from build123d import *

# Parameters (mm, degrees)
SALIENTE_EXTRUIR1_DEPTH = 6


with BuildPart() as part:
    # Croquis1 → Saliente-Extruir1 (new body)
    with BuildSketch(Plane.XY):
        with BuildLine():
            Line((-283.764, 132.5), (-132.5, 132.5))
            Line((-132.5, 132.5), (-132.5, 283.764))
            ThreePointArc((-132.5, 283.764), (-127.012352652, 297.012352652), (-113.764, 302.5))
            Line((-113.764, 302.5), (113.764, 302.5))
            ThreePointArc((113.764, 302.5), (127.012352652, 297.012352652), (132.5, 283.764))
            Line((132.5, 283.764), (132.5, 132.5))
            Line((132.5, 132.5), (283.764, 132.5))
            ThreePointArc((283.764, 132.5), (297.012352652, 127.012352652), (302.5, 113.764))
            Line((302.5, 113.764), (302.5, -113.764))
            ThreePointArc((302.5, -113.764), (297.012352652, -127.012352652), (283.764, -132.5))
            Line((283.764, -132.5), (132.5, -132.5))
            Line((132.5, -132.5), (132.5, -283.764))
            ThreePointArc((132.5, -283.764), (127.012352652, -297.012352652), (113.764, -302.5))
            Line((113.764, -302.5), (-113.764, -302.5))
            ThreePointArc((-113.764, -302.5), (-127.012352652, -297.012352652), (-132.5, -283.764))
            Line((-132.5, -283.764), (-132.5, -132.5))
            Line((-132.5, -132.5), (-283.764, -132.5))
            ThreePointArc((-283.764, -132.5), (-297.012352652, -127.012352652), (-302.5, -113.764))
            Line((-302.5, -113.764), (-302.5, 113.764))
            ThreePointArc((-302.5, 113.764), (-297.012352652, 127.012352652), (-283.764, 132.5))
        make_face()
        with BuildLine():
            Line((-283.764, 122.5), (-122.5, 122.5))
            Line((-122.5, 122.5), (-122.5, 283.764))
            ThreePointArc((-122.5, 283.764), (-119.94128484, 289.94128484), (-113.764, 292.5))
            Line((-113.764, 292.5), (113.764, 292.5))
            ThreePointArc((113.764, 292.5), (119.94128484, 289.94128484), (122.5, 283.764))
            Line((122.5, 283.764), (122.5, 122.5))
            Line((122.5, 122.5), (283.764, 122.5))
            ThreePointArc((283.764, 122.5), (289.94128484, 119.94128484), (292.5, 113.764))
            Line((292.5, 113.764), (292.5, -113.764))
            ThreePointArc((292.5, -113.764), (289.94128484, -119.94128484), (283.764, -122.5))
            Line((283.764, -122.5), (122.5, -122.5))
            Line((122.5, -122.5), (122.5, -283.764))
            ThreePointArc((122.5, -283.764), (119.94128484, -289.94128484), (113.764, -292.5))
            Line((113.764, -292.5), (-113.764, -292.5))
            ThreePointArc((-113.764, -292.5), (-119.94128484, -289.94128484), (-122.5, -283.764))
            Line((-122.5, -283.764), (-122.5, -122.5))
            Line((-122.5, -122.5), (-283.764, -122.5))
            ThreePointArc((-283.764, -122.5), (-289.94128484, -119.94128484), (-292.5, -113.764))
            Line((-292.5, -113.764), (-292.5, 113.764))
            ThreePointArc((-292.5, 113.764), (-289.94128484, 119.94128484), (-283.764, 122.5))
        make_face(mode=Mode.SUBTRACT)
    extrude(amount=SALIENTE_EXTRUIR1_DEPTH)


solid = part.part
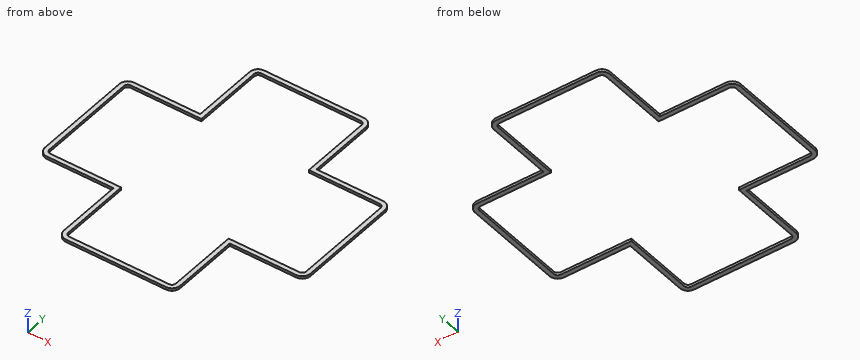
Could you check a few things on this model? Use its own coordinates, in mm. Give positions to 0.01 mm unless a question says otherwise; leave off trailing zeros. Loops run counter-clockwise (first coordinate to the right, second up) from the corner with the lowest first, then second, coordinate; pieces in that order, holes last. Notation, with made-up numbers: (69, 85.5) -> (127, 85.5) arc R15 ccw to (127, 97.5) -> close; hole circle Ø4 at (71.25, 85.5). An arc over 180 degrees is marked (long way). Answer as CSV lines item,"result". Start each with the question number.
(1) If we section it at A-A on y = 204: Write out the boundary of the cut face in (x, z), then the cut area to 3 significant figures.
(2) If we section it at B-B on x = -4.5: Write out the boundary of the cut face in (y, z).
(3) I need wall thicknesses on probe 1 along X at (y, z) = (-225.5, 1.6); probe 2 along X at (y, z) = (-30.5, 4.75). Which ranges of each line are inside material? Lowest first, please.
(4) I'm going to push flat-ended pins straight in: pin 1 Ø3 at (y, z) = (197.5, 1.5) entering from -X; pin 2 Ø3 at (y, z) = (200.5, 4.5) entering from +X; pin 3 Ø1.8 at (x, z) = (-172.5, 2.5) entering from +Y. Where does each tip first touch, or does it pass through?
Computed:
1,outline,"(-132.5, 0) -> (-122.5, 0) -> (-122.5, 6) -> (-132.5, 6) -> close; (122.5, 0) -> (132.5, 0) -> (132.5, 6) -> (122.5, 6) -> close"
1,area,"120 mm2"
2,outline,"(-302.5, 0) -> (-292.5, 0) -> (-292.5, 6) -> (-302.5, 6) -> close; (292.5, 0) -> (302.5, 0) -> (302.5, 6) -> (292.5, 6) -> close"
3,probe 1,"x = -132.5 to -122.5, 122.5 to 132.5"
3,probe 2,"x = -302.5 to -292.5, 292.5 to 302.5"
4,pin 1,"stops at x = -132.5"
4,pin 2,"stops at x = 132.5"
4,pin 3,"stops at y = 132.5"
